Here's how the part is built. I have some questions about the finished solid (model axes, mm). A direction names the side the tool comes from. Round coordinates to 2 decimals unless told otherwise and drop trailing zeros. Write each loop counter-clockwise with the first axis right and the second up, starting at its lowest first coordinate (ties: lowest second). Pieces come first, ordered by that corner, then holes. Notation, with made-up numbers: M 16.25,71 L 38.25,71 A8 ccw 38.25,79 Z; hole C 57.25,47 d8. An arc over 180 degrees is marked long. Write item = value, one per line. Start each with the question number.
(1) I need wall thicknesses on line 1 along Y through (x, z) = (0, 9.3) (1 decimal); line 2 along Y through (x, z) = (9.25, 8.25); line 3 along Z through (x, y) = (2, 8.5). Which ranges of each line are inside material? Lowest first, please.
(2) If we mould it in two halves opening along Y, with no side actions, what happens to faces 1 (the flat face through (-5, -8.3, 8.73)), 2 (the flat face through (6, 0, 11.27)), 3 (the cylindrical face through (5.3, 1.67, 10.8)), 4 (the cylindrical face through (-1.777, 13.536, 5.556))? For each: released by +Y, released by -Y, zero draft, split by the parting line, or undercut.
(3) I want a section at D-D (y = 8.5). List the corners of the cut face in (x, z) for me, and give its area (3 significant figures).
(4) I want a section at C-C (z = 3.5). List the corners of the cut face in (x, y) for me (1 decimal).
(5) On a 3-axis mill with a long thin cutter (end or side, diameter ignored), from which of +Z, -Z, +X, -X, +Y, -Y can I reach the whole of each face in a straight line? I mean faces 5 (the cylindrical face through (10.6, -3.34, 4.3)), 6 (the flat face through (2, -11.1, 0)). Say none if no direction works.
(6) I want a section at B-B (x = -1.5). List the corners of the cut face in (y, z) for me.
(7) I want a section at A-A (y = 0). List the corners of the cut face in (x, z) for me (1 decimal).
(8) Will these pins go through, and if not, where does the flat tip stop? pin 1 Ø11 at (x, y) = (3.5, 0) entering from -Z; pin 2 Ø2 at (x, z) = (5.5, 4) entering from -Y; pin 3 Ø4 at (y, z) = (10, 5) entering from -X.
```python
from build123d import *

# Parameters (mm, degrees)
F0_R     = 13.6525
F1_DEPTH = 11.26998
F2_R     = 11.1125
F3_DEPTH = 8.72998
F4_R     = 9.525
F5_DEPTH = 1.5875
F6_R     = 5.55625
F7_DEPTH = 11.27098


with BuildPart() as f1:
    # F0 (on Top) → F1 (new body)
    with BuildSketch(Plane.XY):
        Circle(F0_R)
    extrude(amount=F1_DEPTH)

    # F2 (on face) → F3 (cut)
    with BuildSketch(Plane(origin=(0, 0, 0), x_dir=(1, 0, 0), z_dir=(0, 0, -1))):
        Circle(F2_R)
    extrude(amount=-F3_DEPTH, mode=Mode.SUBTRACT)

    # F4 (on face) → F5 (cut)
    with BuildSketch(Plane(origin=(0, 0, 8.72998), x_dir=(1, 0, 0), z_dir=(0, 0, -1))):
        Circle(F4_R)
    extrude(amount=-F5_DEPTH, mode=Mode.SUBTRACT)

    # F6 (on face) → F7 (cut, through all)
    with BuildSketch(Plane.XY.offset(11.26998)):
        Circle(F6_R)
    extrude(amount=-F7_DEPTH, mode=Mode.SUBTRACT)


solid = f1.part
```
Returned:
q1.line_1 = -13.7 to -9.5, 9.5 to 13.7
q1.line_2 = -10.04 to -6.16, 6.16 to 10.04
q1.line_3 = 10.32 to 11.27
q2.face_1 = undercut
q2.face_2 = zero draft
q2.face_3 = undercut
q2.face_4 = split by the parting line
q3.outline = M -10.68,0 L -7.16,0 L -7.16,8.73 L -4.3,8.73 L -4.3,10.32 L 4.3,10.32 L 4.3,8.73 L 7.16,8.73 L 7.16,0 L 10.68,0 L 10.68,11.27 L -10.68,11.27 Z
q3.area = 102 mm²
q4.outline = C 0,0 d27.3; hole C 0,0 d22.2
q5.face_5 = -Z
q5.face_6 = -Z, +X, -X, +Y, -Y
q6.outline = M -13.57,0 L -11.01,0 L -11.01,8.73 L -9.41,8.73 L -9.41,10.32 L -5.35,10.32 L -5.35,11.27 L -13.57,11.27 Z; M 5.35,10.32 L 9.41,10.32 L 9.41,8.73 L 11.01,8.73 L 11.01,0 L 13.57,0 L 13.57,11.27 L 5.35,11.27 Z
q7.outline = M -13.7,0 L -11.1,0 L -11.1,8.7 L -9.5,8.7 L -9.5,10.3 L -5.6,10.3 L -5.6,11.3 L -13.7,11.3 Z; M 5.6,10.3 L 9.5,10.3 L 9.5,8.7 L 11.1,8.7 L 11.1,0 L 13.7,0 L 13.7,11.3 L 5.6,11.3 Z
q8.pin_1 = 10.32
q8.pin_2 = -12.89
q8.pin_3 = -11.06
